Verification items for the finished model (mm, model axes). Face numbers are marked on the shaded views. A direction names the side the tool comes from. Coordinates: 2 decimals unless noted, no trailing zeros. Loops run counter-clockwise (first coordinate to the right, second up) from the corner with the lowest first, then second, coordinate; pieces in that order, holes last.
Q1. Mould release check, pull along X, two halves, no side actions. Record for the marked faces 1, 2 and 3: +X half, -X half, draft (parallel to the pull), parting line (faces both ways), or undercut.
Q2. Go/stop test with flat-tipped pins: P1, Ø1, axis at y = 24, z = 18.5, coming from the +X side; P2, Ø6, axis at x = 10.5, z = 42, coming from the -Y side; P3, Ø17, axis at x = 62, y = 29, coming from the +Z side. Record where each tip stops, or that it passes through.
Q3. Material ranges on probe 1 along X at (y, z) = (8.5, 47); probe 2 along Y at (x, z) = (54, 47); probe 3 along Z at (x, y) = (58, 21.5), recorded low to high.
Q4. Sectioned sample at A-A (y = 10). Enter the section's corners in (x, z), then the cut area to 3 significant figures.
Q5. Sectioned sample at B-B (x = 39). Enter the section's corners in (y, z).
Q6. Sectioned sample at C-C (x = 23). Enter the section's corners in (y, z), then the cut area to 3 significant figures.
Q7. Access from +Z, -Z, +X, -X, +Y, -Y to the whole of each face (thin tool, end or side, straight path). Record for the marked faces 4 and 5.
```python
from build123d import *

# Parameters (mm, degrees)
F2_DEPTH = 50.8
F0_W     = 50.8
F0_H     = 38.1
F3_DEPTH = 38.1


with BuildPart() as f2:
    # F1 (on Top) → F2 (new body)
    with BuildSketch(Plane.XY):
        Polygon((0, 50.8), (0, 0), (25.4, 4.233333), (25.4, 38.1), (76.2, 38.1), (76.2, 50.8), align=None)
        Polygon((25.4, 38.1), (25.4, 4.233333), (76.2, 12.7), (76.2, 38.1), align=None)
    extrude(amount=F2_DEPTH)

    # F0 (on Front) → F3 (cut)
    with BuildSketch(Plane.XZ):
        with Locations((50.8, 31.75)):
            Rectangle(F0_W, F0_H)
    extrude(amount=-F3_DEPTH, mode=Mode.SUBTRACT)


solid = f2.part
```
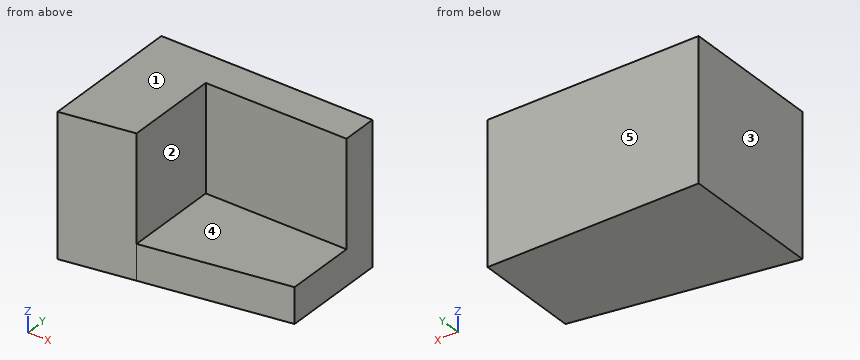
Geometry check:
1. face 1: draft
1. face 2: +X half
1. face 3: -X half
2. P1: stops at x = 25.4
2. P2: stops at y = 1.25
2. P3: stops at z = 12.7
3. probe 1: x = 0 to 25.4
3. probe 2: y = 38.1 to 50.8
3. probe 3: z = 0 to 12.7
4. outline: (0, 0) - (60, 0) - (60, 12.7) - (25.4, 12.7) - (25.4, 50.8) - (0, 50.8) - close
4. area: 1,730 mm2
5. outline: (6.5, 0) - (50.8, 0) - (50.8, 50.8) - (38.1, 50.8) - (38.1, 12.7) - (6.5, 12.7) - close
6. outline: (3.83, 0) - (50.8, 0) - (50.8, 50.8) - (3.83, 50.8) - close
6. area: 2,390 mm2
7. face 4: +Z, +X, -Y
7. face 5: +Z, -Z, +X, -X, +Y
